from build123d import *

# Parameters (mm, degrees)
SKETCH1_W           = 45
SKETCH1_H           = 23
BOSS_EXTRUDE1_DEPTH = 2
SKETCH2_R           = 1.1999976
BOSS_EXTRUDE2_DEPTH = 5
SKETCH3_R           = 1.45
BOSS_EXTRUDE3_DEPTH = 5


with BuildPart() as part:
    # Sketch1 → Boss-Extrude1 (new body)
    with BuildSketch(Plane(origin=(0, 0, 0), x_dir=(1, 0, 0), z_dir=(0, 1, 0))):
        with Locations((22.5, 11.5)):
            Rectangle(SKETCH1_W, SKETCH1_H)
    extrude(amount=-BOSS_EXTRUDE1_DEPTH)

    # Sketch2 → Boss-Extrude2 (add)
    with BuildSketch(Plane(origin=(0, 0, 0), x_dir=(1, 0, 0), z_dir=(0, 1, 0))):
        with Locations((38.8, 2.2)):
            Circle(SKETCH2_R)
    extrude(amount=BOSS_EXTRUDE2_DEPTH)

    # Sketch3 → Boss-Extrude3 (add)
    with BuildSketch(Plane(origin=(0, 0, 0), x_dir=(1, 0, 0), z_dir=(0, 1, 0))):
        with Locations((6.45, 20.5499922)):
            Circle(SKETCH3_R)
    extrude(amount=BOSS_EXTRUDE3_DEPTH)


solid = part.part
Can you work these out from the model? Positions are in its coordinate system, mm. A direction names the side the tool comes from. Coordinates: 2 decimals unless noted, no trailing zeros. Write each loop counter-clockwise with the first axis right and the second up, starting at its lowest first coordinate (ties: lowest second). Pieces come first, ordered by that corner, then holes. Notation, with made-up numbers: (15.25, 14) - (29.25, 14) arc R34 cw to (29.25, 49) - close; hole circle Ø10 at (7.25, -40). An arc over 180 degrees is marked (long way). Return JSON: item names as keys, results as strings. Group by question number.
Item 1: If we section it at C-C (x = 6.45): Write out the boundary of the cut face in (y, z).
Item 2: If we section it at A-A (z = -2.2): Write out the boundary of the cut face in (x, y), then the cut area to 3 significant figures.
Item 3: We'd pull the mould along Y, two halves only. Please class faces 3 (the face through (22, -2, -12)), 4 (the face through (22, -1, -23)), 5 (the face through (39, 5, -2)): pulls with the +Y half, pulls with the -Y half, needs draft (parallel to the pull), parting line crosses it, or undercut.
Item 4: If we section it at B-B (y = 3.25): Write out the boundary of the cut face in (x, z), then the cut area to 3 significant figures.
Item 5: Which directions (+Z, -Z, +X, -X, +Y, -Y) give clear straight access to the entire face, cutting with the end or side of a thin tool? Please do faces 1 (the face through (6, 5, -21)), 2 (the face through (6.136, 2.465, -19.134)).
Item 6: Please list where these lines run through material, in increasing order: probe 1 along Y at (x, z) = (16, -15.25); probe 2 along X at (y, z) = (2.5, -2); probe 3 along X at (y, z) = (4.5, -20).
Item 7: If we section it at D-D (z = -7.5): Write out the boundary of the cut face in (x, y), then the cut area to 3 significant figures.
Item 8: I'm going to push flat-ended pins straight in: pin 1 Ø12 at (x, z) = (18.5, -7) entering from +Y; pin 2 Ø3 at (x, y) = (15, 0.5) entering from -Z. Where does each tip first touch, or does it pass through?
Return value:
{
 "1": {"outline": "(-2, -23) - (0, -23) - (0, -22) - (5, -22) - (5, -19.1) - (0, -19.1) - (0, 0) - (-2, 0) - close"},
 "2": {"outline": "(0, -2) - (45, -2) - (45, 0) - (40, 0) - (40, 5) - (37.6, 5) - (37.6, 0) - (0, 0) - close", "area": "102 mm^2"},
 "3": {"face 3": "pulls with the -Y half", "face 4": "needs draft", "face 5": "pulls with the +Y half"},
 "4": {"outline": "circle Ø2.9 at (6.45, -20.55); circle Ø2.4 at (38.8, -2.2)", "area": "11.1 mm^2"},
 "5": {"face 1": "+Z, -Z, +X, -X, +Y", "face 2": "+Y"},
 "6": {"probe 1": "y = -2 to 0", "probe 2": "x = 37.62 to 39.98", "probe 3": "x = 5.11 to 7.79"},
 "7": {"outline": "(0, -2) - (45, -2) - (45, 0) - (0, 0) - close", "area": "90.0 mm^2"},
 "8": {"pin 1": "stops at y = 0", "pin 2": "stops at z = -23"}
}
